CAD build for the part. Positions are in the model's coordinates, mm. Face numbers are marked on the shaded views. A direction names the side the tool comes from. Coordinates: 2 decimals unless noted, no trailing zeros. Write each loop counter-clockwise with the first axis right and the second up, starting at its lowest first coordinate (ties: lowest second). Pieces come first, ordered by that corner, then holes. Notation, with made-up numbers: (-32, 44.5) - (5, 44.5) arc R26 cw to (5, 62.5) - close; hole circle Ø2 at (59.25, -16.75). An arc over 180 degrees is marked (long way). One line per question, with ' | ' between items. Start each with the question number.
1. Band-saw the part on B-B, the plane y = 3.75. Write the cut outline in (x, z).
2. Band-saw the part on C-C, the plane z = 18. Write the cut outline in (x, y).
3. Band-saw the part on A-A, the plane y = -2.5. Write the cut outline in (x, z), then the cut area to 3 significant figures.
4. Band-saw the part on D-D, the plane x = -8.5. Write the cut outline in (y, z).
5. Probe line 1 (X direction, y = 2.5, z = 12.75); line 2 (X direction, y = -2.25, z = 9.5); line 3 (Y direction, x = 0, z = 3). List the from-to ranges inside material, lowest first.
6. Flat gauge pins, fed straight in: P1, Ø1.7, axis at x = -33, z = 13, coming from the -Y side; P2, Ø2, axis at x = -22, z = 10.5, coming from the +Y side. Where does each tip first touch, or does it go through?
7. Which spindle directions (+Z, -Z, +X, -X, +Y, -Y) get a long thin tool onto all of the face, cutting with end or side? Do the marked faces 1, 2 and 3. Say none if no direction does.
Autodesk Fusion 360 part; units mm, degrees
sketch "Sketch1" plane through (0, 0, 0) normal (0, 0, 1) x (1, 0, 0)
  line L0 (-40.65, 0) -> (40.65, 0)
  line L1 (40.65, 0) -> (40.65, 13)
  line L2 (40.65, 13) -> (0, 8)
  line L3 (0, 8) -> (-40.65, 13)
  line L4 (-40.65, 13) -> (-40.65, 0)
  line L5 (0, 8) -> (0, 0) construction
  dimension "d1" = 13
  dimension "d2" = 8
  dimension "d3" = 81.3
extrude "Extrude1" add sketch "Sketch1" along normal blind 22
sketch "Sketch2" plane through (0, 0, 0) normal (0, 0, -1) x (-1, 0, 0)
  line L0 (40.65, 0) -> (40.65, 13)
  line L1 (40.65, 13) -> (0, 8)
  line L2 (0, 8) -> (-40.65, 13)
  line L3 (-40.65, 13) -> (-40.65, 0)
  line L4 (-40.65, 0) -> (40.65, 0)
  line L5 (24.05, 4.5) -> (31.05, 4.5)
  line L6 (31.05, 4.5) -> (31.05, 0)
  line L7 (31.05, 0) -> (24.05, 0)
  line L8 (24.05, 0) -> (24.05, 4.5)
  line L9 (18.6, 10.2878) -> (18.6, 0) construction
  line L10 (36.5, 12.4895) -> (36.5, 0)
  line L11 (0, 8) -> (0, 0) construction
  line L12 (-24.05, 0) -> (-24.05, 4.5)
  line L13 (-24.05, 4.5) -> (-31.05, 4.5)
  line L14 (-31.05, 0) -> (-24.05, 0)
  line L15 (-31.05, 4.5) -> (-31.05, 0)
  point P0 (27.55, 0)
  dimension "d7" = 7
  dimension "d9" = 8.95
  dimension "d10" = 4.5
  dimension "d11" = 4.15
  dimension "d12" = 17.9
extrude "Extrude2" cut sketch "Sketch2" against normal blind 22 contours L4 L5 L6 L7 L8 | L4 L12 L13 L14 L15
sketch "Sketch3" plane through (0, 0, 0) normal (0, 0, -1) x (-1, 0, 0)
  line L0 (31.05, 4.5) -> (31.05, 0)
  line L1 (31.05, 0) -> (40.65, 0)
  line L2 (40.65, 0) -> (40.65, 13)
  line L3 (40.65, 13) -> (0, 8)
  line L4 (0, 8) -> (-40.65, 13)
  line L5 (-40.65, 13) -> (-40.65, 0)
  line L6 (-40.65, 0) -> (-31.05, 0)
  line L7 (-31.05, 0) -> (-31.05, 4.5)
  line L8 (-31.05, 4.5) -> (-24.05, 4.5)
  line L9 (-24.05, 4.5) -> (-24.05, 0)
  line L10 (-24.05, 0) -> (24.05, 0)
  line L11 (24.05, 0) -> (24.05, 4.5)
  line L12 (24.05, 4.5) -> (31.05, 4.5)
  line L13 (0, 8) -> (0, 0) construction
  line L14 (40.65, 0) -> (36.65, 0)
  line L15 (36.65, 0) -> (36.65, -6)
  line L16 (36.65, -6) -> (40.65, -6)
  line L17 (40.65, -6) -> (40.65, 0)
  line L18 (-36.65, 0) -> (-36.65, -6)
  line L19 (-36.65, -6) -> (-40.65, -6)
  line L20 (-40.65, 0) -> (-36.65, 0)
  line L21 (-40.65, -6) -> (-40.65, 0)
  dimension "d15" = 4
  dimension "d16" = 6
extrude "Extrude3" add sketch "Sketch3" against normal blind 22 contours L1 L14 L15 L16 L17 | L6 L18 L19 L20 L21
fillet "Fillet1" radius 4 2 edges at (-40.65, 13, 11) (40.65, 13, 11)
fillet "Fillet2" radius 2 2 edges at (40.65, -6, 11) (-40.65, -6, 11)
equation "d3 = 73 mm + 2 * tolerance + ( 2 * 4 ) * 1 mm"
equation "tolerance = 0.15 mm"
equation "d9 = ( 17.9 / 2 ) * 1 mm"
equation "d11 = 4 mm + tolerance"
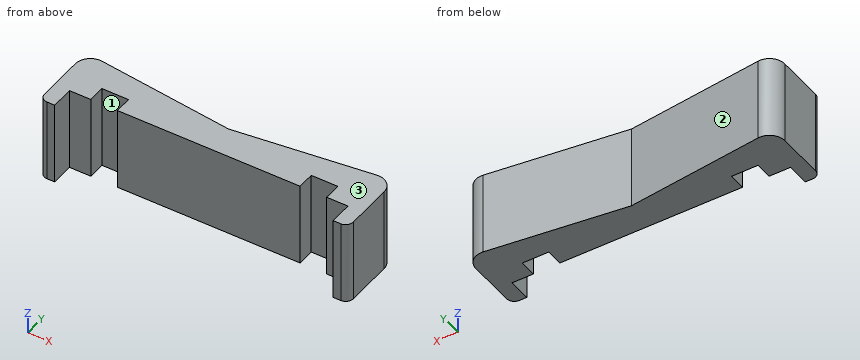
Filled in:
1) outline: (-40.65, 0) - (-31.05, 0) - (-31.05, 22) - (-40.65, 22) - close; (-24.05, 0) - (24.05, 0) - (24.05, 22) - (-24.05, 22) - close; (31.05, 0) - (40.65, 0) - (40.65, 22) - (31.05, 22) - close
2) outline: (-40.65, -4) arc R2 ccw to (-38.65, -6) - (-36.65, -6) - (-36.65, 0) - (-31.05, 0) - (-31.05, 4.5) - (-24.05, 4.5) - (-24.05, 0) - (24.05, 0) - (24.05, 4.5) - (31.05, 4.5) - (31.05, 0) - (36.65, 0) - (36.65, -6) - (38.65, -6) arc R2 ccw to (40.65, -4) - (40.65, 8.48) arc R4 ccw to (36.16, 12.45) - (0, 8) - (-36.16, 12.45) arc R4 ccw to (-40.65, 8.48) - close
3) outline: (-40.65, 0) - (-36.65, 0) - (-36.65, 22) - (-40.65, 22) - close; (36.65, 0) - (40.65, 0) - (40.65, 22) - (36.65, 22) - close | area: 176 mm²
4) outline: (0, 0) - (9.05, 0) - (9.05, 22) - (0, 22) - close
5) line 1: x = -40.65 to -31.05, -24.05 to 24.05, 31.05 to 40.65 | line 2: x = -40.65 to -36.65, 36.65 to 40.65 | line 3: y = 0 to 8
6) P1: stops at y = 0 | P2: stops at y = 10.83
7) face 1: +Z, -Z, -Y | face 2: +Z, -Z, +Y | face 3: +Z, +X, -X, +Y, -Y
